Could you check a few things on this model? Use its own coordinates, in mm. A direction names the side the tool comes from. Round coordinates to 2 decimals unless told otherwise and drop trailing zeros. Loops run counter-clockwise (first coordinate to the right, second up) from the corner with the lowest first, then second, coordinate; pieces in that order, holes last. Notation, with made-up numbers: (75.5, 29.25) - (92.5, 29.25) arc R17 cw to (92.5, 58.25) - close; hole circle Ø9 at (55, -26). An arc over 180 degrees is marked (long way). Answer as CSV lines item,"result". Start each with the question number.
1) Suppose I cut it at B-B, the plane x = 52.5. Write out the boundary of the cut face in (y, z).
2) We'd pull the mould along X, two halves only. Please class faces 3 (the face through (81.6, 28.5, -36.7)), 4 (the face through (0, 17, -44)), 5 (the face through (76.05, 33.146, -88.045)): pulls with the +X half, pulls with the -X half, needs draft (parallel to the pull), parting line crosses it, or undercut.
3) I'm going to push flat-ended pins straight in: pin 1 Ø3 at (x, z) = (38, -57.5) entering from -Y; pin 2 Ø1.5 at (y, z) = (17.5, -60) entering from +X; pin 3 Ø4 at (y, z) = (7, -72) entering from +X. Where does each tip first touch, or does it pass through?
4) Please list where these lines run through material, in increasing order: line 1 along Y through (x, z) = (123, -60.5); line 2 along X through (y, z) = (30, -64); line 3 along Z through (x, y) = (126, 12.5).
5) Which directions (+Z, -Z, +X, -X, +Y, -Y) give clear straight access to the entire face, cutting with the end or side of a thin tool? Please do faces 1 (the face through (76.05, 33.045, -1.854)), 2 (the face through (85.5, 20, -64)).
6) Suppose I cut it at A-A, the plane y = 4. Count the separate pieces of the cut face and the enclosed holes in it, then the cut area to 3 significant figures.
```python
from build123d import *

# Parameters (mm, degrees)
SKETCH1_W             = 150
SKETCH1_H             = 90
BOSS_EXTRUDE1_DEPTH   = 35
SHELL2_T              = -2.5
SKETCH5_R             = 4
BOSS_EXTRUDE8_DEPTH   = 32.5
SKETCH6_R             = 1.25
CUT_EXTRUDE1_DEPTH    = 12
SKETCH6_3_R           = 1.25
CUT_EXTRUDE2_DEPTH    = 12
FILLET1_R             = 6.5
FILLET2_R             = 6.5
SKETCH22_R            = 3
SKETCH22_R_2          = 1.25
ESP32_SCREWHOLE_DEPTH = 4
SKETCH25_R            = 3
SKETCH25_R_2          = 1.25
BOSS_EXTRUDE11_DEPTH  = 4
GUIDE_HW_DEPTH        = 5
BOSS_EXTRUDE13_DEPTH  = 16.5
SKETCH33_W            = 23
SKETCH33_H            = 2
BOSS_EXTRUDE14_DEPTH  = 10
SKETCH36_R            = 9.5
CUT_EXTRUDE8_DEPTH    = 2
CUT_EXTRUDE9_START    = -2
SKETCH37_R            = 9.5
CUT_EXTRUDE9_DEPTH    = 2
SKETCH38_R            = 7.5
SKETCH38_R_2          = 3.05
BOSS_EXTRUDE15_DEPTH  = 10
SKETCH40_W            = 1.5
SKETCH40_H            = 15
CUT_EXTRUDE10_DEPTH   = 2.5
SKETCH41_W            = 12
SKETCH41_H            = 7
CUT_EXTRUDE11_DEPTH   = 2.5
SKETCH42_W            = 12
SKETCH42_H            = 7
CUT_EXTRUDE12_DEPTH   = 2.5
SKETCH45_W            = 2
SKETCH45_H            = 32
BOSS_EXTRUDE16_DEPTH  = 25
SKETCH47_R            = 3
CUT_EXTRUDE13_DEPTH   = 2.5
SKETCH43_R            = 10.25
SKETCH43_R_2          = 8.75
BOSS_EXTRUDE18_DEPTH  = 45


with BuildPart() as part:
    # Sketch1 → Boss-Extrude1 (new body)
    with BuildSketch(Plane(origin=(0, 0, 0), x_dir=(1, 0, 0), z_dir=(0, 1, 0))):
        with Locations((75, 45)):
            Rectangle(SKETCH1_W, SKETCH1_H)
    extrude(amount=BOSS_EXTRUDE1_DEPTH)

    # Shell2
    shell2_openings = [part.faces().sort_by_distance(p)[0] for p in [
        (75, 0, -45),
    ]]
    offset(amount=SHELL2_T, openings=shell2_openings, kind=Kind.INTERSECTION)

    # Sketch5 → Boss-Extrude8 (add)
    with BuildSketch(Plane(origin=(0, 32.5, 0), x_dir=(-1, 0, 0), z_dir=(0, -1, 0))):
        with Locations(Location((-8.5, 81.5, 0), (0, 0, 90))):
            Circle(SKETCH5_R)
        with Locations(Location((-8.5, 8.5, 0), (0, 0, 90))):
            Circle(SKETCH5_R)
        with Locations(Location((-141.5, 81.5, 0), (0, 0, 90))):
            Circle(SKETCH5_R)
        with Locations(Location((-141.5, 8.5, 0), (0, 0, 90))):
            Circle(SKETCH5_R)
    extrude(amount=BOSS_EXTRUDE8_DEPTH)

    # Sketch6 → Cut-Extrude1 (cut)
    with BuildSketch(Plane.XZ):
        with Locations(Location((8.5, -81.5, 0), (0, 0, 270))):
            Circle(SKETCH6_R)
    extrude(amount=-CUT_EXTRUDE1_DEPTH, mode=Mode.SUBTRACT)

    # Sketch6_3 → Cut-Extrude2 (cut)
    with BuildSketch(Plane.XZ):
        with Locations(Location((141.5, -81.5, 0), (0, 0, 270))):
            Circle(SKETCH6_3_R)
        with Locations(Location((141.5, -8.5, 0), (0, 0, 270))):
            Circle(SKETCH6_3_R)
        with Locations(Location((8.5, -8.5, 0), (0, 0, 270))):
            Circle(SKETCH6_3_R)
    extrude(amount=-CUT_EXTRUDE2_DEPTH, mode=Mode.SUBTRACT)

    # Fillet1
    fillet1_edges = [part.edges().sort_by_distance(p)[0] for p in [
        (75, 35, 0),
    ]]
    fillet(fillet1_edges, radius=FILLET1_R)

    # Fillet2
    fillet2_edges = [part.edges().sort_by_distance(p)[0] for p in [
        (75, 35, -90),
    ]]
    fillet(fillet2_edges, radius=FILLET2_R)

    # Sketch22 → ESP32-screwhole (add)
    # profile 1 of 4: a face of its own
    with BuildSketch(Plane.XZ.offset(-32.5)):
        with Locations(Location((82.9, -36.1, 0), (0, 0, 270))):
            Circle(SKETCH22_R)
        with Locations(Location((82.9, -36.1, 0), (0, 0, 270))):
            Circle(SKETCH22_R_2, mode=Mode.SUBTRACT)
    # profile 2 of 4: a face of its own
    with BuildSketch(Plane.XZ.offset(-32.5)):
        with Locations(Location((82.9, -9.9, 0), (0, 0, 270))):
            Circle(SKETCH22_R)
        with Locations(Location((82.9, -9.9, 0), (0, 0, 270))):
            Circle(SKETCH22_R_2, mode=Mode.SUBTRACT)
    # profile 3 of 4: a face of its own
    with BuildSketch(Plane.XZ.offset(-32.5)):
        with Locations(Location((131.1, -9.9, 0), (0, 0, 270))):
            Circle(SKETCH22_R)
        with Locations(Location((131.1, -9.9, 0), (0, 0, 270))):
            Circle(SKETCH22_R_2, mode=Mode.SUBTRACT)
    # profile 4 of 4: a face of its own
    with BuildSketch(Plane.XZ.offset(-32.5)):
        with Locations(Location((131.1, -36.1, 0), (0, 0, 270))):
            Circle(SKETCH22_R)
        with Locations(Location((131.1, -36.1, 0), (0, 0, 270))):
            Circle(SKETCH22_R_2, mode=Mode.SUBTRACT)
    extrude(amount=ESP32_SCREWHOLE_DEPTH)

    # Sketch25 → Boss-Extrude11 (add)
    # profile 1 of 4: a face of its own
    with BuildSketch(Plane.XZ.offset(-32.5)):
        with Locations(Location((6, -70.5, 0), (0, 0, 270))):
            Circle(SKETCH25_R)
        with Locations(Location((6, -70.5, 0), (0, 0, 270))):
            Circle(SKETCH25_R_2, mode=Mode.SUBTRACT)
    # profile 2 of 4: a face of its own
    with BuildSketch(Plane.XZ.offset(-32.5)):
        with Locations(Location((6, -57.5, 0), (0, 0, 270))):
            Circle(SKETCH25_R)
        with Locations(Location((6, -57.5, 0), (0, 0, 270))):
            Circle(SKETCH25_R_2, mode=Mode.SUBTRACT)
    # profile 3 of 4: a face of its own
    with BuildSketch(Plane.XZ.offset(-32.5)):
        with Locations(Location((38, -57.5, 0), (0, 0, 270))):
            Circle(SKETCH25_R)
        with Locations(Location((38, -57.5, 0), (0, 0, 270))):
            Circle(SKETCH25_R_2, mode=Mode.SUBTRACT)
    # profile 4 of 4: a face of its own
    with BuildSketch(Plane.XZ.offset(-32.5)):
        with Locations(Location((38, -70.5, 0), (0, 0, 270))):
            Circle(SKETCH25_R)
        with Locations(Location((38, -70.5, 0), (0, 0, 270))):
            Circle(SKETCH25_R_2, mode=Mode.SUBTRACT)
    extrude(amount=BOSS_EXTRUDE11_DEPTH)

    # Sketch30 → guide HW (add)
    with BuildSketch(Plane.XZ.offset(-32.5)):
        Polygon((2.5, -52), (28.1, -52), (28.1, -32.4), (2.5, -32.4), (2.5, -30.9), (29.6, -30.9), (29.6, -53.5), (2.5, -53.5), align=None)
    extrude(amount=GUIDE_HW_DEPTH)

    # Sketch32 → Boss-Extrude13 (add)
    with BuildSketch(Plane.XZ.offset(-32.5)):
        Polygon((2.5, -29.4), (8.9, -29.4), (8.9, -16.2), (2.5, -16.2), (2.5, -14.7), (10.4, -14.7), (10.4, -30.9), (2.5, -30.9), align=None)
    extrude(amount=BOSS_EXTRUDE13_DEPTH)

    # Sketch33 → Boss-Extrude14 (add)
    with BuildSketch(Plane.XZ.offset(-32.5)):
        with Locations((57.5, -76.5)):
            Rectangle(SKETCH33_W, SKETCH33_H)
        with Locations((57.5, -11.5)):
            Rectangle(SKETCH33_W, SKETCH33_H)
    extrude(amount=BOSS_EXTRUDE14_DEPTH)

    # Sketch36 → Cut-Extrude8 (cut)
    with BuildSketch(Plane.XY.offset(-75.5)):
        with Locations((57.5, 22.5)):
            Circle(SKETCH36_R)
    extrude(amount=-CUT_EXTRUDE8_DEPTH, mode=Mode.SUBTRACT)

    # Sketch37 → Cut-Extrude9 (cut)
    with BuildSketch(Plane(origin=(0, 0, -12.5), x_dir=(-1, 0, 0), z_dir=(0, 0, -1)).offset(CUT_EXTRUDE9_START)):
        with Locations((-57.5, 22.5)):
            Circle(SKETCH37_R)
    extrude(amount=CUT_EXTRUDE9_DEPTH, mode=Mode.SUBTRACT)

    # Sketch38 → Boss-Extrude15 (add)
    with BuildSketch(Plane(origin=(150, 0, 0), x_dir=(0, 0, -1), z_dir=(1, 0, 0))):
        with Locations((60.5, 18)):
            Circle(SKETCH38_R)
        with Locations((60.5, 18)):
            Circle(SKETCH38_R_2, mode=Mode.SUBTRACT)
    extrude(amount=BOSS_EXTRUDE15_DEPTH)

    # Sketch40 → Cut-Extrude10 (cut)
    with BuildSketch(Plane.ZY):
        with Locations((-28.65, 24)):
            Rectangle(SKETCH40_W, SKETCH40_H)
        with Locations((-25.65, 24)):
            Rectangle(SKETCH40_W, SKETCH40_H)
        with Locations((-22.65, 24)):
            Rectangle(SKETCH40_W, SKETCH40_H)
        with Locations((-19.65, 24)):
            Rectangle(SKETCH40_W, SKETCH40_H)
        with Locations((-16.65, 24)):
            Rectangle(SKETCH40_W, SKETCH40_H)
    extrude(amount=-CUT_EXTRUDE10_DEPTH, mode=Mode.SUBTRACT)

    # Sketch41 → Cut-Extrude11 (cut)
    with BuildSketch(Plane.ZY):
        with Locations((-41.7, 26.5)):
            Rectangle(SKETCH41_W, SKETCH41_H)
    extrude(amount=-CUT_EXTRUDE11_DEPTH, mode=Mode.SUBTRACT)

    # Sketch42 → Cut-Extrude12 (cut)
    with BuildSketch(Plane.ZY):
        with Locations((-64, 24)):
            Rectangle(SKETCH42_W, SKETCH42_H)
    extrude(amount=-CUT_EXTRUDE12_DEPTH, mode=Mode.SUBTRACT)

    # Sketch45 → Boss-Extrude16 (add)
    with BuildSketch(Plane.XZ.offset(-32.5)):
        with Locations((86.5, -63.5)):
            Rectangle(SKETCH45_W, SKETCH45_H)
    extrude(amount=BOSS_EXTRUDE16_DEPTH)

    # Sketch47 → Cut-Extrude13 (cut)
    with BuildSketch(Plane.ZY.offset(-147.5)):
        with Locations((-60.5, 18)):
            Circle(SKETCH47_R)
    extrude(amount=-CUT_EXTRUDE13_DEPTH, mode=Mode.SUBTRACT)

    # Sketch43 → Boss-Extrude18 (add)
    with BuildSketch(Plane.ZY.offset(-147.5)):
        with Locations(Location((-60.5, 18, 0), (0, 0, 180))):
            Circle(SKETCH43_R)
        with Locations(Location((-60.5, 18, 0), (0, 0, 180))):
            Circle(SKETCH43_R_2, mode=Mode.SUBTRACT)
    extrude(amount=BOSS_EXTRUDE18_DEPTH)


solid = part.part
```
Filled sheet:
1,outline,"(0, -90) - (28.5, -90) arc R6.5 ccw to (35, -83.5) - (35, -6.5) arc R6.5 ccw to (28.5, 0) - (0, 0) - (0, -2.5) - (32.5, -2.5) - (32.5, -10.5) - (30.58, -10.5) - (30.58, -12.5) - (32.5, -12.5) - (32.5, -75.5) - (30.58, -75.5) - (30.58, -77.5) - (32.5, -77.5) - (32.5, -87.5) - (0, -87.5) - close"
2,face 3,"undercut"
2,face 4,"pulls with the -X half"
2,face 5,"needs draft"
3,pin 1,"y = 28.5"
3,pin 2,"x = 87.5"
3,pin 3,"x = 150"
4,line 1,"7.75 to 9.25, 26.75 to 28.25, 32.5 to 35"
4,line 2,"0 to 2.5, 85.5 to 87.5, 147.5 to 150"
4,line 3,"-90 to -87.5, -69.15 to -67.31, -53.69 to -51.85, -2.5 to 0"
5,face 1,"+Z, +X, -X, +Y"
5,face 2,"-Y"
6,separate pieces,"5"
6,enclosed holes,"5"
6,area,"1,360 mm²"
